Can you work these out from the model? Positions are in its coordinate system, mm. A direction names the side the tool comes from. Coordinates: 2 decimals unless noted, no trailing zeros. Order: outer loops, then holes, each group sorted by start corner. A loop starts at its lowest first (then second) coordinate and runs counter-clockwise, first axis right, second up. Notation, with made-up numbers: (24.25, 85) -> (61.25, 85) arc R9 cw to (61.25, 92) -> close; hole circle Ø7 at (66, 51). An arc over 180 degrees is marked (long way). Use a Markdown table: item, result. Add a question column.
1. Suppose I cut it at C-C, the plane y = -15. State how many separate pieces and enclosed holes the cut face has, then the cut area to 3 significant figures.
2. We'd pull the mould along X, two halves only. Please class faces 4 (the flat face through (0, -101.6, -6)), 5 (the cylindrical face through (-35.713, -68.517, 40.564)): pulls with the +X half, pulls with the -X half, needs draft (parallel to the pull), parting line crosses it, or undercut.
3. For pin 1 Ø6 at (x, y) = (-33.02, -43.87) entering from +Z; pin 2 Ø11 at (x, y) = (-35, -14.5) entering from -Z; pin 3 Ø8 at (x, z) = (24, 14) entering from +Y; pin 4 Ø6 at (x, y) = (0, -72.73) entering from +Z, each with a flat end and sliding along its axis, tell me the tip position at first contact or that it passes through.
4. Suppose I cut it at D-D, the plane x = 44. List the corners of the cut face in (y, z) for me.
5. If I drill on line 1 along Z through (x, y) = (0, 12); line 2 along Y through (x, z) = (41, -1.5); line 3 along Y through (x, z) = (-32.5, 39), over which ranges is the centre line in solid material (lowest first)? Write a range as from..to.
6. Suppose I cut it at A-A, the plane x = 24. List the corners of the cut face in (y, z) for me, then the cut area to 3 significant figures.
7. Suppose I cut it at B-B, the plane z = -21. List the corners of the cut face in (x, y) for me.
8. For faces 1 (the flat face through (-37, 0, 43)), 2 (the flat face through (38, 0, 44)), 3 (the flat face through (31, -46, 43.175)), which set-ups out of +Z, -Z, +X, -X, +Y, -Y let a thin tool reach every point of the face, with its end or its side?
```python
from build123d import *

# Parameters (mm, degrees)
SKETCH1_R               = 50.8
SKETCH1_R_2             = 38.1
BOSS_EXTRUDE1_DEPTH     = 20
SKETCH2_W               = 31.907935637
SKETCH2_H               = 10.300850003
BOSS_EXTRUDE2_DEPTH     = 101.6
BOSS_EXTRUDE3_DEPTH     = 101.6
SKETCH4_R               = 50.816877582
BOSS_EXTRUDE4_DEPTH     = 10
SKETCH6_W               = 34.862909764
SKETCH6_H               = 101.6
BOSS_EXTRUDE5_DEPTH     = 10
SKETCH7_W               = 34.862909764
SKETCH7_H               = 101.6
BOSS_EXTRUDE6_DEPTH     = 10
SKETCH8_R               = 2.5
CUT_EXTRUDE1_DEPTH      = 3.870178859
CUT_EXTRUDE1_DEPTH_BACK = 99.824625306
SKETCH10_R              = 5
CUT_EXTRUDE2_DEPTH      = 5.15
SKETCH11_R              = 2.5
CUT_EXTRUDE3_DEPTH      = 3.870178859
CUT_EXTRUDE3_DEPTH_BACK = 99.824625306
SKETCH12_R              = 5
CUT_EXTRUDE4_DEPTH      = 5.15
SKETCH13_R              = 2.5
CUT_EXTRUDE5_DEPTH      = 89.824625306
CUT_EXTRUDE5_DEPTH_BACK = 13.870178859
SKETCH14_R              = 5
CUT_EXTRUDE6_DEPTH      = 5.15


with BuildPart() as part:
    # Sketch1 → Boss-Extrude1 (new body)
    with BuildSketch(Plane(origin=(0, 0, 0), x_dir=(1, 0, 0), z_dir=(0, 1, 0))):
        Circle(SKETCH1_R)
        Circle(SKETCH1_R_2, mode=Mode.SUBTRACT)
    extrude(amount=BOSS_EXTRUDE1_DEPTH)

    # Sketch2 → Boss-Extrude2 (add)
    with BuildSketch(Plane.XZ):
        with Locations((0.29228093, 43.175050308)):
            Rectangle(SKETCH2_W, SKETCH2_H)
    extrude(amount=BOSS_EXTRUDE2_DEPTH)

    # Sketch3 → Boss-Extrude3 (add)
    with BuildSketch(Plane.XZ.offset(101.6)):
        with BuildLine():
            Line((-15.661686888, 48.325475309), (16.246248749, 48.325475309))
            ThreePointArc((16.246248749, 48.325475309), (0.292280931, 50.894804165), (-15.661686888, 48.325475309))
        make_face()
    extrude(amount=-BOSS_EXTRUDE3_DEPTH)

    # Sketch4 → Boss-Extrude4 (add)
    with BuildSketch(Plane.XZ.offset(101.6)):
        with Locations((0.292280931, 0.077926583)):
            Circle(SKETCH4_R)
    extrude(amount=BOSS_EXTRUDE4_DEPTH)

    # Sketch6 → Boss-Extrude5 (add)
    with BuildSketch(Plane(origin=(0, 0, 38.024625306), x_dir=(-1, 0, 0), z_dir=(0, 0, -1))):
        with Locations((33.09314177, -50.8)):
            Rectangle(SKETCH6_W, SKETCH6_H)
    extrude(amount=-BOSS_EXTRUDE5_DEPTH)

    # Sketch7 → Boss-Extrude6 (add)
    with BuildSketch(Plane(origin=(0, 0, 38.024625306), x_dir=(-1, 0, 0), z_dir=(0, 0, -1))):
        with Locations((-33.677703631, -50.8)):
            Rectangle(SKETCH7_W, SKETCH7_H)
    extrude(amount=-BOSS_EXTRUDE6_DEPTH)

    # Sketch8 → Cut-Extrude1 (cut, two sides)
    with BuildSketch(Plane.XY.offset(48.024625306)) as cut_extrude1_sk:
        with Locations((33.609158513, -15)):
            Circle(SKETCH8_R)
        with Locations((33.609158513, -43.86666666)):
            Circle(SKETCH8_R)
        with Locations((33.609158513, -72.733333333)):
            Circle(SKETCH8_R)
    extrude(amount=CUT_EXTRUDE1_DEPTH, mode=Mode.SUBTRACT)
    extrude(cut_extrude1_sk.sketch, amount=-CUT_EXTRUDE1_DEPTH_BACK, mode=Mode.SUBTRACT)

    # Sketch10 → Cut-Extrude2 (cut)
    with BuildSketch(Plane(origin=(0, 0, 38.024625306), x_dir=(-1, 0, 0), z_dir=(0, 0, -1))):
        with Locations((-33.609158513, -15)):
            Circle(SKETCH10_R)
        with Locations((-33.609158513, -43.86666666)):
            Circle(SKETCH10_R)
        with Locations((-33.609158513, -72.733333333)):
            Circle(SKETCH10_R)
    extrude(amount=-CUT_EXTRUDE2_DEPTH, mode=Mode.SUBTRACT)

    # Sketch11 → Cut-Extrude3 (cut, two sides)
    with BuildSketch(Plane.XY.offset(48.024625306)) as cut_extrude3_sk:
        with Locations((-33.024596652, -15)):
            Circle(SKETCH11_R)
        with Locations((-33.024596652, -43.866666667)):
            Circle(SKETCH11_R)
        with Locations((-33.024596652, -72.733333333)):
            Circle(SKETCH11_R)
    extrude(amount=CUT_EXTRUDE3_DEPTH, mode=Mode.SUBTRACT)
    extrude(cut_extrude3_sk.sketch, amount=-CUT_EXTRUDE3_DEPTH_BACK, mode=Mode.SUBTRACT)

    # Sketch12 → Cut-Extrude4 (cut)
    with BuildSketch(Plane(origin=(0, 0, 38.024625306), x_dir=(-1, 0, 0), z_dir=(0, 0, -1))):
        with Locations((33.024596652, -15)):
            Circle(SKETCH12_R)
        with Locations((33.024596652, -43.866666667)):
            Circle(SKETCH12_R)
        with Locations((33.024596652, -72.733333333)):
            Circle(SKETCH12_R)
    extrude(amount=-CUT_EXTRUDE4_DEPTH, mode=Mode.SUBTRACT)

    # Sketch13 → Cut-Extrude5 (cut, two sides)
    with BuildSketch(Plane(origin=(0, 0, 38.024625306), x_dir=(-1, 0, 0), z_dir=(0, 0, -1))) as cut_extrude5_sk:
        with Locations((-1.549603414, -15)):
            Circle(SKETCH13_R)
        with Locations((0, -43.866666667)):
            Circle(SKETCH13_R)
        with Locations((0, -72.733333333)):
            Circle(SKETCH13_R)
    extrude(amount=CUT_EXTRUDE5_DEPTH, mode=Mode.SUBTRACT)
    extrude(cut_extrude5_sk.sketch, amount=-CUT_EXTRUDE5_DEPTH_BACK, mode=Mode.SUBTRACT)

    # Sketch14 → Cut-Extrude6 (cut)
    with BuildSketch(Plane(origin=(0, 0, 38.024625306), x_dir=(-1, 0, 0), z_dir=(0, 0, -1))):
        with Locations((-1.549603414, -15)):
            Circle(SKETCH14_R)
        with Locations((0, -43.866666667)):
            Circle(SKETCH14_R)
        with Locations((0, -72.733333333)):
            Circle(SKETCH14_R)
    extrude(amount=-CUT_EXTRUDE6_DEPTH, mode=Mode.SUBTRACT)


solid = part.part
```
Worked out:
| question | item | result |
|---|---|---|
| 1 | separate pieces | 4 |
| 1 | enclosed holes | 0 |
| 1 | area | 839 mm² |
| 2 | face 4 | needs draft |
| 2 | face 5 | undercut |
| 3 | pin 1 | stops at z = 48.02 |
| 3 | pin 2 | stops at z = 38.02 |
| 3 | pin 3 | stops at y = -101.6 |
| 3 | pin 4 | stops at z = 50.89 |
| 4 | outline | (-111.6, -25.84) -> (-101.6, -25.84) -> (-101.6, 26) -> (-111.6, 26) -> close; (-101.6, 38.02) -> (0, 38.02) -> (0, 48.02) -> (-101.6, 48.02) -> close; (0, -25.39) -> (20, -25.39) -> (20, 25.39) -> (0, 25.39) -> close |
| 5 | line 1 | z = -50.8..-38.1, 38.1..50.8 |
| 5 | line 2 | y = -111.6..-101.6, 0..20 |
| 5 | line 3 | y = -101.6..-77.71, -67.76..-48.84, -38.89..-19.97, -10.03..20 |
| 6 | outline | (-111.6, -44.87) -> (-101.6, -44.87) -> (-101.6, 38.02) -> (0, 38.02) -> (0, 29.59) -> (20, 29.59) -> (20, 44.77) -> (0, 44.77) -> (0, 48.02) -> (-101.6, 48.02) -> (-101.6, 45.03) -> (-111.6, 45.03) -> close; (0, -44.77) -> (20, -44.77) -> (20, -29.59) -> (0, -29.59) -> close |
| 6 | area | 2,520 mm² |
| 7 | outline | (-46.26, 0) -> (-31.79, 0) -> (-31.79, 20) -> (-46.26, 20) -> close; (-45.95, -111.6) -> (46.53, -111.6) -> (46.53, -101.6) -> (-45.95, -101.6) -> close; (31.79, 0) -> (46.26, 0) -> (46.26, 20) -> (31.79, 20) -> close |
| 8 | face 1 | +Z, -X, +Y |
| 8 | face 2 | +Z, +X, +Y |
| 8 | face 3 | -Z |
